The listing builds one solid part. Answer for the finished solid, in the listing's coordinates (mm). A direction names the side the tool comes from. Round coordinates to 2 decimals unless told otherwise and drop trailing zeros. Order: outer loops, then holes, each group sorted by start corner. A loop starts at its lowest first (then second) coordinate and runs counter-clockwise, first axis right, second up. Notation, with made-up numbers: (60, -18.5) - (71, -18.5) arc R7 cw to (71, -5.5) - close; hole circle Ø3 at (-14, 62). An arc over 180 degrees is marked (long way). One line per item, written item: value. Start each with the question number.
1. Flat-ended cylindrical pins translate along their axes: P1, Ø1, axis at y = -1, z = -1.5, coming from the +X side; P2, Ø5.5, axis at y = -4.5, z = -18, coming from the -X side; P3, Ø8, axis at x = 73, z = 23.5, coming from the +Y side. Find the tip coordinate at first contact, or state that the pin passes through.
2. Straight lines are drawn through the part: line 1 (X direction, y = 2.75, z = 50); line 2 (X direction, y = -1, z = -42.5); line 3 (Z direction, x = 4.5, y = 9). For each, find the intervals that lie inside material, in ascending order.
3. Section D-D, the plane z = -18 is taken. Give the vertices of the cut face in (x, y), then the cut area to 3 significant figures.
4. Section B-B, the plane z = -50 is taken. Give the vertices of the cut face in (x, y).
5. Section A-A, the plane x = -90 is taken. Give the vertices of the cut face in (y, z), then the cut area to 3 significant figures.
6. Section C-C, the plane y = 6 is taken. Give the vertices of the cut face in (x, z), then the cut area to 3 significant figures.
7. For a pull along X with two mould halves and no side action, classify faces 4 (the flat face through (-88, 0, -1)), 5 (the flat face through (-100, 5, 1)), 6 (the flat face through (80, 7, 1)), 7 (the flat face through (-1, 7, -40)) as released by +X, released by -X, zero draft, split by the parting line, or undercut.
8. A tool of negligible diameter and unlimited length cuts with its end or side. For faces 1 (the flat face through (-25, -4, -15)), 2 (the flat face through (-20, -3, 18)), 3 (the flat face through (-25, -3, 20)), from which of +Z, -Z, +X, -X, +Y, -Y can it reach the whole face along a straight path? Write none if from no direction.
from build123d import *

# Parameters (mm, degrees)
SKETCH1_W             = 200
SKETCH1_H             = 120
BOSS_EXTRUDE3_DEPTH   = 10
SKETCH3_R             = 3.75
SKETCH3_W             = 160
SKETCH3_H             = 80
CUT_EXTRUDE2_DEPTH    = 6
SKETCH6_R             = 3.75
CUT_EXTRUDE4_DEPTH    = 117.773284616
SKETCH7_W             = 30
SKETCH7_H             = 120
BOSS_EXTRUDE4_DEPTH   = 2
SKETCH8_W             = 10
SKETCH8_H             = 5
BOSS_EXTRUDE5_DEPTH   = 2
BOSS_EXTRUDE5_2_DEPTH = 2
BOSS_EXTRUDE5_3_DEPTH = 2
BOSS_EXTRUDE5_4_DEPTH = 2
SKETCH10_W            = 10
SKETCH10_H            = 5
BOSS_EXTRUDE6_DEPTH   = 5


with BuildPart() as part:
    # Sketch1 → Boss-Extrude3 (new body)
    with BuildSketch(Plane(origin=(0, 0, 0), x_dir=(1, 0, 0), z_dir=(0, 1, 0))):
        Rectangle(SKETCH1_W, SKETCH1_H)
    extrude(amount=BOSS_EXTRUDE3_DEPTH)

    # Sketch3 → Cut-Extrude2 (cut)
    with BuildSketch(Plane(origin=(0, 10, 0), x_dir=(1, 0, 0), z_dir=(0, 1, 0))):
        with Locations(Location((-90, 50, 0), (0, 0, 270))):
            Circle(SKETCH3_R)
        with Locations(Location((90, -50, 0), (0, 0, 270))):
            Circle(SKETCH3_R)
        with Locations(Location((90, 50, 0), (0, 0, 270))):
            Circle(SKETCH3_R)
        with Locations(Location((-90, -50, 0), (0, 0, 270))):
            Circle(SKETCH3_R)
        Rectangle(SKETCH3_W, SKETCH3_H)
    extrude(amount=-CUT_EXTRUDE2_DEPTH, mode=Mode.SUBTRACT)

    # Sketch6 → Cut-Extrude4 (cut, through all)
    with BuildSketch(Plane(origin=(0, 4, 0), x_dir=(1, 0, 0), z_dir=(0, 1, 0))):
        with Locations(Location((-90, 50, 0), (0, 0, 270))):
            Circle(SKETCH6_R)
        with Locations(Location((90, 50, 0), (0, 0, 270))):
            Circle(SKETCH6_R)
        with Locations(Location((90, -50, 0), (0, 0, 270))):
            Circle(SKETCH6_R)
        with Locations(Location((-90, -50, 0), (0, 0, 270))):
            Circle(SKETCH6_R)
    extrude(amount=-CUT_EXTRUDE4_DEPTH, mode=Mode.SUBTRACT)

    # Sketch7 → Boss-Extrude4 (add)
    with BuildSketch(Plane(origin=(0, 0, 0), x_dir=(-1, 0, 0), z_dir=(0, -1, 0))):
        Rectangle(SKETCH7_W, SKETCH7_H)
        with Locations((60, 0)):
            Rectangle(SKETCH7_W, SKETCH7_H)
        with Locations((-60, 0)):
            Rectangle(SKETCH7_W, SKETCH7_H)
    extrude(amount=BOSS_EXTRUDE4_DEPTH)



with BuildPart() as body_2:
    # Sketch8 → Boss-Extrude5 (new body)
    with BuildSketch(Plane(origin=(0, -2, 0), x_dir=(-1, 0, 0), z_dir=(0, -1, 0))):
        with Locations((25, -17.5)):
            Rectangle(SKETCH8_W, SKETCH8_H)
    extrude(amount=-BOSS_EXTRUDE5_DEPTH)


with BuildPart() as body_3:
    # Sketch8 → Boss-Extrude5 2 (new body)
    with BuildSketch(Plane(origin=(0, -2, 0), x_dir=(-1, 0, 0), z_dir=(0, -1, 0))):
        with Locations((-25, -17.5)):
            Rectangle(SKETCH8_W, SKETCH8_H)
    extrude(amount=-BOSS_EXTRUDE5_2_DEPTH)


with BuildPart() as body_4:
    # Sketch8 → Boss-Extrude5 3 (new body)
    with BuildSketch(Plane(origin=(0, -2, 0), x_dir=(-1, 0, 0), z_dir=(0, -1, 0))):
        with Locations((-25, 17.5)):
            Rectangle(SKETCH8_W, SKETCH8_H)
    extrude(amount=-BOSS_EXTRUDE5_3_DEPTH)


with BuildPart() as body_5:
    # Sketch8 → Boss-Extrude5 4 (new body)
    with BuildSketch(Plane(origin=(0, -2, 0), x_dir=(-1, 0, 0), z_dir=(0, -1, 0))):
        with Locations((25, 17.5)):
            Rectangle(SKETCH8_W, SKETCH8_H)
    extrude(amount=-BOSS_EXTRUDE5_4_DEPTH)


with BuildPart() as part_1:
    add(part.part)

    add(body_2.part)  # Boss-Extrude6 merges body 2

    add(body_3.part)  # Boss-Extrude6 merges body 3

    add(body_4.part)  # Boss-Extrude6 merges body 4

    add(body_5.part)  # Boss-Extrude6 merges body 5
    # Sketch10 → Boss-Extrude6 (add)
    with BuildSketch(Plane(origin=(0, -2, 0), x_dir=(-1, 0, 0), z_dir=(0, -1, 0))):
        with Locations((25, -17.5)):
            Rectangle(SKETCH10_W, SKETCH10_H)
        with Locations((25, 17.5)):
            Rectangle(SKETCH10_W, SKETCH10_H)
        with Locations((-25, 17.5)):
            Rectangle(SKETCH10_W, SKETCH10_H)
        with Locations((-25, -17.5)):
            Rectangle(SKETCH10_W, SKETCH10_H)
    extrude(amount=BOSS_EXTRUDE6_DEPTH)


solid = part_1.part
Answer list:
1. P1: stops at x = 75
1. P2: stops at x = -75
1. P3: stops at y = 4
2. line 1: x = -100 to -93.75, -86.25 to 86.25, 93.75 to 100
2. line 2: x = -75 to -45, -15 to 15, 45 to 75
2. line 3: z = -60 to -40, 40 to 60
3. outline: (-100, 0) - (-75, 0) - (-75, -2) - (-45, -2) - (-45, 0) - (-30, 0) - (-30, -7) - (-20, -7) - (-20, 0) - (-15, 0) - (-15, -2) - (15, -2) - (15, 0) - (20, 0) - (20, -7) - (30, -7) - (30, 0) - (45, 0) - (45, -2) - (75, -2) - (75, 0) - (100, 0) - (100, 10) - (80, 10) - (80, 4) - (-80, 4) - (-80, 10) - (-100, 10) - close
3. area: 1,360 mm²
4. outline: (-100, 0) - (-93.75, 0) - (-93.75, 10) - (-100, 10) - close; (-86.25, 0) - (-75, 0) - (-75, -2) - (-45, -2) - (-45, 0) - (-15, 0) - (-15, -2) - (15, -2) - (15, 0) - (45, 0) - (45, -2) - (75, -2) - (75, 0) - (86.25, 0) - (86.25, 10) - (-86.25, 10) - close; (93.75, 0) - (100, 0) - (100, 10) - (93.75, 10) - close
5. outline: (0, -60) - (10, -60) - (10, -53.75) - (0, -53.75) - close; (0, -46.25) - (10, -46.25) - (10, 46.25) - (0, 46.25) - close; (0, 53.75) - (10, 53.75) - (10, 60) - (0, 60) - close
5. area: 1,050 mm²
6. outline: (-100, -60) - (100, -60) - (100, 60) - (-100, 60) - close; hole circle Ø7.5 at (-90, -50); hole circle Ø7.5 at (-90, 50); hole (-80, -40) - (80, -40) - (80, 40) - (-80, 40) - close; hole circle Ø7.5 at (90, -50); hole circle Ø7.5 at (90, 50)
6. area: 11,000 mm²
7. face 4: zero draft
7. face 5: released by -X
7. face 6: undercut
7. face 7: undercut
8. face 1: -Y
8. face 2: +Z, -Z, -Y
8. face 3: +Z, -Y
